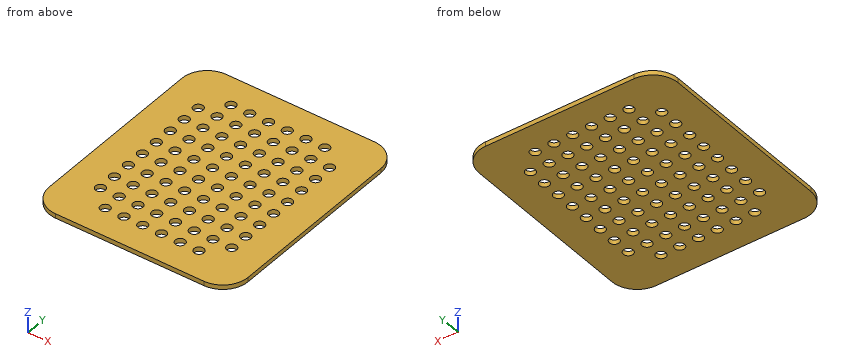
from build123d import *

# Parameters (mm, degrees)
F1_DEPTH      = 1.5
F3_R          = 1.65
F4_DEPTH      = 12.2
F4_DEPTH_BACK = 25


with BuildPart() as f1:
    # F0 (on Top) → F1 (new body)
    with BuildSketch(Plane.XY):
        with BuildLine():
            ThreePointArc((33.4, 29.9), (30.910408, 35.910408), (24.9, 38.4))
            Line((24.9, 38.4), (-24.9, 38.4))
            ThreePointArc((-24.9, 38.4), (-30.910408, 35.910408), (-33.4, 29.9))
            Line((-33.4, 29.9), (-33.4, -29.9))
            ThreePointArc((-33.4, -29.9), (-30.910408, -35.910408), (-24.9, -38.4))
            Line((-24.9, -38.4), (24.9, -38.4))
            ThreePointArc((24.9, -38.4), (30.910408, -35.910408), (33.4, -29.9))
            Line((33.4, -29.9), (33.4, 29.9))
        make_face()
    extrude(amount=F1_DEPTH)

    # F3 (on face) → F4 (cut, two sides)
    with BuildSketch(Plane.XY.offset(1.5)) as f4_sk:
        with Locations((-22.05, 22.05)):
            Circle(F3_R)
        with Locations((-22.05, 15.75)):
            Circle(F3_R)
        with Locations((-22.05, 9.45)):
            Circle(F3_R)
        with Locations((-22.05, 3.15)):
            Circle(F3_R)
        with Locations((-22.05, -3.15)):
            Circle(F3_R)
        with Locations((-22.05, -9.45)):
            Circle(F3_R)
        with Locations((-22.05, -15.75)):
            Circle(F3_R)
        with Locations((-22.05, -22.05)):
            Circle(F3_R)
        with Locations((-15.75, 28.35)):
            Circle(F3_R)
        with Locations((-15.75, 22.05)):
            Circle(F3_R)
        with Locations((-15.75, 15.75)):
            Circle(F3_R)
        with Locations((-15.75, 9.45)):
            Circle(F3_R)
        with Locations((-15.75, 3.15)):
            Circle(F3_R)
        with Locations((-15.75, -3.15)):
            Circle(F3_R)
        with Locations((-15.75, -9.45)):
            Circle(F3_R)
        with Locations((-15.75, -15.75)):
            Circle(F3_R)
        with Locations((-15.75, -22.05)):
            Circle(F3_R)
        with Locations((-15.75, -28.35)):
            Circle(F3_R)
        with Locations((-9.45, 28.35)):
            Circle(F3_R)
        with Locations((-9.45, 22.05)):
            Circle(F3_R)
        with Locations((-9.45, 15.75)):
            Circle(F3_R)
        with Locations((-9.45, 9.45)):
            Circle(F3_R)
        with Locations((-9.45, 3.15)):
            Circle(F3_R)
        with Locations((-9.45, -3.15)):
            Circle(F3_R)
        with Locations((-9.45, -9.45)):
            Circle(F3_R)
        with Locations((-9.45, -15.75)):
            Circle(F3_R)
        with Locations((-9.45, -22.05)):
            Circle(F3_R)
        with Locations((-9.45, -28.35)):
            Circle(F3_R)
        with Locations((-3.15, 28.35)):
            Circle(F3_R)
        with Locations((-3.15, 22.05)):
            Circle(F3_R)
        with Locations((-3.15, 15.75)):
            Circle(F3_R)
        with Locations((-3.15, 9.45)):
            Circle(F3_R)
        with Locations((-3.15, 3.15)):
            Circle(F3_R)
        with Locations((-3.15, -3.15)):
            Circle(F3_R)
        with Locations((-3.15, -9.45)):
            Circle(F3_R)
        with Locations((-3.15, -15.75)):
            Circle(F3_R)
        with Locations((-3.15, -22.05)):
            Circle(F3_R)
        with Locations((-3.15, -28.35)):
            Circle(F3_R)
        with Locations((3.15, 28.35)):
            Circle(F3_R)
        with Locations((3.15, 22.05)):
            Circle(F3_R)
        with Locations((3.15, 15.75)):
            Circle(F3_R)
        with Locations((3.15, 9.45)):
            Circle(F3_R)
        with Locations((3.15, 3.15)):
            Circle(F3_R)
        with Locations((3.15, -3.15)):
            Circle(F3_R)
        with Locations((3.15, -9.45)):
            Circle(F3_R)
        with Locations((3.15, -15.75)):
            Circle(F3_R)
        with Locations((3.15, -22.05)):
            Circle(F3_R)
        with Locations((3.15, -28.35)):
            Circle(F3_R)
        with Locations((9.45, 28.35)):
            Circle(F3_R)
        with Locations((9.45, 22.05)):
            Circle(F3_R)
        with Locations((9.45, 15.75)):
            Circle(F3_R)
        with Locations((9.45, 9.45)):
            Circle(F3_R)
        with Locations((9.45, 3.15)):
            Circle(F3_R)
        with Locations((9.45, -3.15)):
            Circle(F3_R)
        with Locations((9.45, -9.45)):
            Circle(F3_R)
        with Locations((9.45, -15.75)):
            Circle(F3_R)
        with Locations((9.45, -22.05)):
            Circle(F3_R)
        with Locations((9.45, -28.35)):
            Circle(F3_R)
        with Locations((15.75, 28.35)):
            Circle(F3_R)
        with Locations((15.75, 22.05)):
            Circle(F3_R)
        with Locations((15.75, 15.75)):
            Circle(F3_R)
        with Locations((15.75, 9.45)):
            Circle(F3_R)
        with Locations((15.75, 3.15)):
            Circle(F3_R)
        with Locations((15.75, -3.15)):
            Circle(F3_R)
        with Locations((15.75, -9.45)):
            Circle(F3_R)
        with Locations((15.75, -15.75)):
            Circle(F3_R)
        with Locations((15.75, -22.05)):
            Circle(F3_R)
        with Locations((15.75, -28.35)):
            Circle(F3_R)
        with Locations((22.05, 22.05)):
            Circle(F3_R)
        with Locations((22.05, 15.75)):
            Circle(F3_R)
        with Locations((22.05, 9.45)):
            Circle(F3_R)
        with Locations((22.05, 3.15)):
            Circle(F3_R)
        with Locations((22.05, -3.15)):
            Circle(F3_R)
        with Locations((22.05, -9.45)):
            Circle(F3_R)
        with Locations((22.05, -15.75)):
            Circle(F3_R)
        with Locations((22.05, -22.05)):
            Circle(F3_R)
    extrude(amount=-F4_DEPTH, mode=Mode.SUBTRACT)
    extrude(f4_sk.sketch, amount=-F4_DEPTH_BACK, mode=Mode.SUBTRACT)


solid = f1.part
Could you check a few things on this model? Use its own coordinates, in mm. Coordinates: 2 decimals unless noted, no trailing zeros. Order: outer loops, then holes, each group sorted by start corner. A loop starts at its lowest first (then second) coordinate and runs counter-clockwise, first axis right, second up.
Q1. Will this pin go through, and if not, where does the flat tip stop? pin 1 (2 mm diameter, centred on x = 3.15, y = -9.45, fed in from -Z).
Q2. Please list where these lines run through material, in increasing order: L1, parallel to Y at x = -28, z = 1.35; L2, parallel to Y at x = 30, z = 0.7.
Q3. Suppose I cut it at B-B on x = -22.05. Give the number of separate pieces and of enclosed holes in the cut face, and give its area (3 significant figures).
Q4. Suppose I cut it at A-A on y = -28.35. Please give me the cut outline in (x, z).
Answer:
1. pin 1: passes through
2. L1: y = -37.81 to 37.81
2. L2: y = -36.7 to 36.7
3. separate pieces: 9
3. enclosed holes: 0
3. area: 75.6 mm2
4. outline: (-33.4, 0) - (-17.4, 0) - (-17.4, 1.5) - (-33.4, 1.5) - close; (-14.1, 0) - (-11.1, 0) - (-11.1, 1.5) - (-14.1, 1.5) - close; (-7.8, 0) - (-4.8, 0) - (-4.8, 1.5) - (-7.8, 1.5) - close; (-1.5, 0) - (1.5, 0) - (1.5, 1.5) - (-1.5, 1.5) - close; (4.8, 0) - (7.8, 0) - (7.8, 1.5) - (4.8, 1.5) - close; (11.1, 0) - (14.1, 0) - (14.1, 1.5) - (11.1, 1.5) - close; (17.4, 0) - (33.4, 0) - (33.4, 1.5) - (17.4, 1.5) - close
